from build123d import *

# Parameters (mm, degrees)
SKETCH1_W               = 12.7
SKETCH1_H               = 28.575
BOSS_EXTRUDE1_DEPTH     = 111.76
SKETCH3_W               = 1.397
SKETCH3_H               = 28.575
BOSS_EXTRUDE3_DEPTH     = 15.748
SKETCH7_R               = 1.27
CUT_EXTRUDE3_DEPTH      = 1
CUT_EXTRUDE3_DEPTH_BACK = 13.7


with BuildPart() as part:
    # Sketch1 → Boss-Extrude1 (new body)
    with BuildSketch(Plane.XY):
        with Locations((6.35, 14.2875)):
            Rectangle(SKETCH1_W, SKETCH1_H)
    extrude(amount=BOSS_EXTRUDE1_DEPTH)

    # Sketch3 → Boss-Extrude3 (add)
    with BuildSketch(Plane(origin=(0, 0, 0), x_dir=(-1, 0, 0), z_dir=(0, 0, -1))):
        with Locations((-0.6985, 14.2875)):
            Rectangle(SKETCH3_W, SKETCH3_H)
        with Locations((-12.0015, 14.2875)):
            Rectangle(SKETCH3_W, SKETCH3_H)
    extrude(amount=BOSS_EXTRUDE3_DEPTH)

    # Sketch7 → Cut-Extrude3 (cut, two sides)
    with BuildSketch(Plane.ZY) as cut_extrude3_sk:
        with Locations((-13.208, 25.0952)):
            Circle(SKETCH7_R)
        with Locations((-2.54, 2.54)):
            Circle(SKETCH7_R)
    extrude(amount=CUT_EXTRUDE3_DEPTH, mode=Mode.SUBTRACT)
    extrude(cut_extrude3_sk.sketch, amount=-CUT_EXTRUDE3_DEPTH_BACK, mode=Mode.SUBTRACT)


solid = part.part
Build history of the part. All positions in model axes, mm. A direction names the side the tool comes from. Coordinates: 2 decimals unless noted, no trailing zeros. Order: outer loops, then holes, each group sorted by start corner. A loop starts at its lowest first (then second) coordinate and runs counter-clockwise, first axis right, second up. Notation, with made-up numbers: (-6.75, 56) -> (41.25, 56) arc R20 cw to (41.25, 85) -> close; hole circle Ø9 at (-23.75, 32.5). An arc over 180 degrees is marked (long way). One line per item, written item: value.
(1) Mould opens along Y. For faces 3 (the flat face through (6, 14, 0)), 4 (the flat face through (6, 28.575, 49)), 5 (the cylindrical face through (0.689, 26.354, -13.373)) say: pulls with the +Y half, pulls with the -Y half, needs draft (parallel to the pull), parting line crosses it, or undercut.
Checked values:
face 3: needs draft
face 4: pulls with the +Y half
face 5: undercut
(2) Probe line 1 (Y direction, x = 0.8, z = -2.54) (3 decimals); line 2 (Z direction, x = 3.75, y = 19.25). List the from-to ranges inside material, lowest first. Write a range as [from, to].
Checked values:
line 1: [0, 1.27], [3.81, 28.575]
line 2: [0, 111.76]
(3) Slice it at D-D, the plane x = 4.5. List the corners of the cut face in (y, z) (3 decimals), plus the area to 3 significant figures.
Checked values:
outline: (0, 0) -> (28.575, 0) -> (28.575, 111.76) -> (0, 111.76) -> close
area: 3,190 mm2
(4) Drop flat-ended pins along their axis: pin 1 Ø5 at (x, z) = (6, 96.5) entering from -Y; pin 2 Ø5 at (x, y) = (7.5, 12) entering from -Z. Give the stop position or say it passes through.
Checked values:
pin 1: y = 0
pin 2: z = 0
(5) Slice it at B-B, the plane y = 2.54. List the corners of the cut face in (x, z), plus the area to 3 significant figures.
Checked values:
outline: (0, -15.75) -> (1.4, -15.75) -> (1.4, -3.81) -> (0, -3.81) -> close; (0, -1.27) -> (1.4, -1.27) -> (1.4, 0) -> (11.3, 0) -> (11.3, -1.27) -> (12.7, -1.27) -> (12.7, 111.76) -> (0, 111.76) -> close; (11.3, -15.75) -> (12.7, -15.75) -> (12.7, -3.81) -> (11.3, -3.81) -> close
area: 1,460 mm2
(6) Slice it at C-C, the plane y = 21.5. List the corners of the cut face in (x, z), plus the area to 3 significant figures.
Checked values:
outline: (0, -15.75) -> (1.4, -15.75) -> (1.4, 0) -> (11.3, 0) -> (11.3, -15.75) -> (12.7, -15.75) -> (12.7, 111.76) -> (0, 111.76) -> close
area: 1,460 mm2
(7) Slice it at A-A, the plane z = -2.54. List the corners of the cut face in (x, y) (3 decimals), plus the area to 3 significant figures.
Checked values:
outline: (0, 0) -> (1.397, 0) -> (1.397, 1.27) -> (0, 1.27) -> close; (0, 3.81) -> (1.397, 3.81) -> (1.397, 28.575) -> (0, 28.575) -> close; (11.303, 0) -> (12.7, 0) -> (12.7, 1.27) -> (11.303, 1.27) -> close; (11.303, 3.81) -> (12.7, 3.81) -> (12.7, 28.575) -> (11.303, 28.575) -> close
area: 72.7 mm2
(8) Tool access for faces 1 (the flat face through (1.397, 14, -8)), 2 (the flat face through (6, 14, 111.76)): list every direction of +Z, -Z, +X, -X, +Y, -Y with a clear straight run to the whole face (end or side of a thin tool).
Checked values:
face 1: -Z, +Y, -Y
face 2: +Z, +X, -X, +Y, -Y
